Read the model definition and answer for the solid it produces. Units are mm, in the model's axes. Face numbers are marked on the shaded views. Coordinates: 2 decimals unless noted, no trailing zeros. Write each loop counter-clockwise with the first axis right and the second up, starting at its lowest first coordinate (ties: lowest second). Pieces come first, ordered by that corner, then holes. Notation, with made-up numbers: (23.25, 73.25) -> (50.25, 73.25) arc R11 ccw to (50.25, 83.25) -> close; hole circle Ø1 at (73, 63). An arc over 180 degrees is marked (long way). Use CSV: the item, a comma, the result in double quotes.
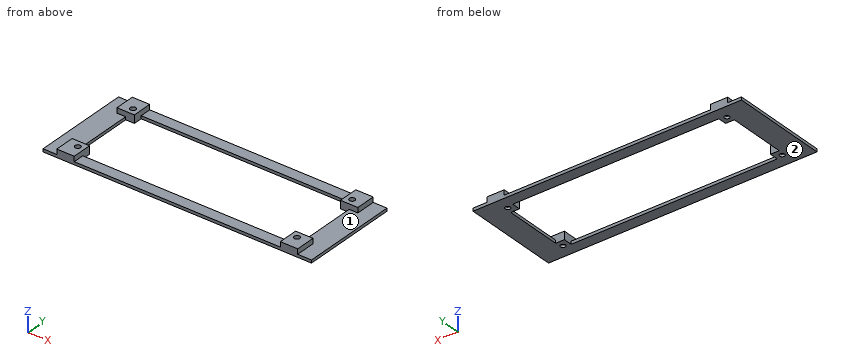
from build123d import *

# Parameters (mm, degrees)
SKICA1_W                                          = 185
SKICA1_H                                          = 67
SKICA1_W_2                                        = 154
SKICA1_H_2                                        = 51.8
SKICA1_W_3                                        = 6
SKICA1_H_3                                        = 6
P_IDAT_VYSUNUT_M1_DEPTH                           = 2
SKICA2_W                                          = 12
SKICA2_H                                          = 13.6
P_IDAT_VYSUNUT_M2_DEPTH                           = 3.5
V_LCOV_ZAHLOUBEN_PRO_M3_ROUBY_S_HLAVO_D           = 3.4
V_LCOV_ZAHLOUBEN_PRO_M3_ROUBY_S_HLAVO_CBORE_D     = 3.8
V_LCOV_ZAHLOUBEN_PRO_M3_ROUBY_S_HLAVO_CBORE_DEPTH = 4


with BuildPart() as part:
    # Skica1 → Přidat vysunutím1 (new body)
    with BuildSketch(Plane.XY):
        Rectangle(SKICA1_W, SKICA1_H)
        Rectangle(SKICA1_W_2, SKICA1_H_2, mode=Mode.SUBTRACT)
        with Locations((-74, 22.9)):
            Rectangle(SKICA1_W_3, SKICA1_H_3)
        with Locations((-74, -22.9)):
            Rectangle(SKICA1_W_3, SKICA1_H_3)
        with Locations((74, -22.9)):
            Rectangle(SKICA1_W_3, SKICA1_H_3)
        with Locations((74, 22.9)):
            Rectangle(SKICA1_W_3, SKICA1_H_3)
    extrude(amount=P_IDAT_VYSUNUT_M1_DEPTH)

    # Skica2 → Přidat vysunutím2 (add)
    with BuildSketch(Plane.XY.offset(2)):
        with Locations((77, 26.7)):
            Rectangle(SKICA2_W, SKICA2_H)
        with Locations((-77, 26.7)):
            Rectangle(SKICA2_W, SKICA2_H)
        with Locations((-77, -26.7)):
            Rectangle(SKICA2_W, SKICA2_H)
        with Locations((77, -26.7)):
            Rectangle(SKICA2_W, SKICA2_H)
    extrude(amount=P_IDAT_VYSUNUT_M2_DEPTH)

    # Válcové zahloubení pro M3 šrouby s hlavou s vnitřním vybráním1 (through all)
    with Locations(Plane.XY.offset(5.5)):
        with Locations((75.5, -24.5), (75.5, 24.5), (-75.5, 24.5), (-75.5, -24.5)):
            CounterBoreHole(V_LCOV_ZAHLOUBEN_PRO_M3_ROUBY_S_HLAVO_D / 2, V_LCOV_ZAHLOUBEN_PRO_M3_ROUBY_S_HLAVO_CBORE_D / 2, V_LCOV_ZAHLOUBEN_PRO_M3_ROUBY_S_HLAVO_CBORE_DEPTH)


solid = part.part
1. A cutting plane is placed at B-B (x = 53.5). Give the vertices of the cut face in (y, z), and give its area (3 significant figures).
Solutions:
outline,"(-33.5, 0) -> (-25.9, 0) -> (-25.9, 2) -> (-33.5, 2) -> close; (25.9, 0) -> (33.5, 0) -> (33.5, 2) -> (25.9, 2) -> close"
area,"30.4 mm^2"
2. This flat-tipped pin is pushed along its axis until it touches: pin 1 Ø4 at (x, y) = (-15, -29) entering from +Z. Where does it stop, or does it pass through?
Solutions:
pin 1,"stops at z = 2"
3. Find the intervals of material crossed by line 1 along Y through (x, z) = (-75.5, 0.9); line 2 along Y through (x, z) = (-75.5, 3.85); line 3 along Y through (x, z) = (72.5, 5.25), in increasing order.
Solutions:
line 1,"y = -33.5 to -26.2, -22.8 to -19.9, 19.9 to 22.8, 26.2 to 33.5"
line 2,"y = -33.5 to -26.4, -22.6 to -19.9, 19.9 to 22.6, 26.4 to 33.5"
line 3,"y = -33.5 to -19.9, 19.9 to 33.5"
4. For a pull along Y with two mould halves and no side action, classify the marked faces 1 and 2 as pulls with the +Y half, pulls with the -Y half, needs draft (parallel to the pull), parting line crosses it, or undercut.
Solutions:
face 1,"undercut"
face 2,"needs draft"
5. A cutting plane is placed at C-C (y = -3). Give the vertices of the cut face in (x, z).
Solutions:
outline,"(-92.5, 0) -> (-77, 0) -> (-77, 2) -> (-92.5, 2) -> close; (77, 0) -> (92.5, 0) -> (92.5, 2) -> (77, 2) -> close"
6. A cutting plane is placed at A-A (z = 4.05). Give the vertices of the cut face in (x, y).
Solutions:
outline,"(-83, -33.5) -> (-71, -33.5) -> (-71, -19.9) -> (-83, -19.9) -> close; (-83, 19.9) -> (-71, 19.9) -> (-71, 33.5) -> (-83, 33.5) -> close; (71, -33.5) -> (83, -33.5) -> (83, -19.9) -> (71, -19.9) -> close; (71, 19.9) -> (83, 19.9) -> (83, 33.5) -> (71, 33.5) -> close; hole circle Ø3.8 at (-75.5, -24.5); hole circle Ø3.8 at (-75.5, 24.5); hole circle Ø3.8 at (75.5, -24.5); hole circle Ø3.8 at (75.5, 24.5)"
